from build123d import *

# Parameters (mm, degrees)
BOSS_EXTRUDE1_DEPTH = 10
SKETCH4_W           = 60
SKETCH4_H           = 60
BOSS_EXTRUDE2_DEPTH = 10
SKETCH5_W           = 60
SKETCH5_H           = 147
BOSS_EXTRUDE3_DEPTH = 8
SKETCH6_R           = 12.5
CUT_EXTRUDE1_DEPTH  = 72
SKETCH7_R           = 12.5
BOSS_EXTRUDE4_DEPTH = 50


with BuildPart() as part:
    # Sketch2 → Boss-Extrude1 (new body)
    with BuildSketch(Plane.XY.offset(30)):
        with BuildLine():
            Line((0, -80), (30, -80))
            Line((30, -80), (30, 10))
            Line((30, 10), (15, 77))
            ThreePointArc((15, 77), (-7.5, 92.648353456), (-30, 77))
            Line((-30, 77), (-30, -80))
            Line((-30, -80), (0, -80))
        make_face()
    boss_extrude1 = extrude(amount=BOSS_EXTRUDE1_DEPTH)

    # Sketch4 → Boss-Extrude2 (add)
    with BuildSketch(Plane.XZ.offset(80)):
        Rectangle(SKETCH4_W, SKETCH4_H)
    extrude(amount=-BOSS_EXTRUDE2_DEPTH)

    # Mirror3: Boss-Extrude1 across plane
    add(boss_extrude1.mirror(Plane.XY))

    # Sketch5 → Boss-Extrude3 (add)
    with BuildSketch(Plane.ZY.offset(30)):
        with Locations((0, 3.5)):
            Rectangle(SKETCH5_W, SKETCH5_H)
    extrude(amount=-BOSS_EXTRUDE3_DEPTH)

    # Sketch6 → Cut-Extrude1 (cut, symmetric)
    with BuildSketch(Plane.XY):
        with Locations(Location((0, 0, 0), (0, 0, 180))):
            Circle(SKETCH6_R)
    extrude(amount=CUT_EXTRUDE1_DEPTH, both=True, mode=Mode.SUBTRACT)

    # Sketch7 → Boss-Extrude4 (add)
    with BuildSketch(Plane.XZ.offset(80)):
        with Locations(Location((0, 0, 0), (0, 0, 270))):
            Circle(SKETCH7_R)
    extrude(amount=BOSS_EXTRUDE4_DEPTH)


solid = part.part
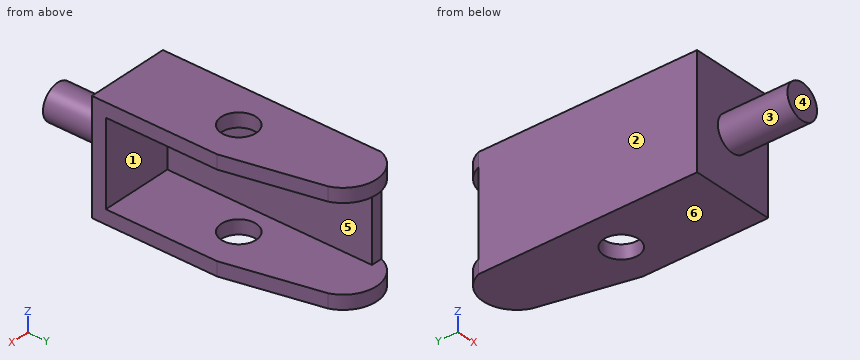
Read the model definition and answer for the solid it produces. Units are mm, in the model's axes. Face numbers are marked on the shaded views. A direction names the side the tool comes from. Coordinates: 2 decimals unless noted, no trailing zeros. Loops run counter-clockwise (first coordinate to the right, second up) from the corner with the lowest first, then second, coordinate; pieces in that order, holes last.
Q1. Each of these flat-tipped pins is pushed along its axis until it touches: pin 1 Ø1 at (x, z) = (-9, 25.5) entering from +Y; pin 2 Ø2 at (y, z) = (-55.5, 16) entering from +X; pin 3 Ø12 at (x, z) = (-6.5, -21) entering from -Y. Where does it stop, or does it pass through?
Q2. Which of the six approach directions +Z, -Z, +X, -X, +Y, -Y give full straight-line access (tool end or side, diameter ignored) to the marked faces 1, 2 and 3?
Q3. The part is cut by section B-B on z = 0. Write down the section's boundary in (x, y), and give its area (3 significant figures).
Q4. The part is cut by section A-A on y = 0. Write down the section's boundary in (x, z).
Q5. The mould has two halves that part along Z. Classify the marked faces 4, 5 and 6: +Z half, -Z half, draft (parallel to the pull), parting line (faces both ways), or undercut.
Q6. The part is cut by section C-C on x = 0. Write down the section's boundary in (y, z), and give its area (3 significant figures).
Q7. Consider probe 1 along Z at (x, y) = (-15.5, 57.5); probe 2 along X at (y, z) = (33.5, 1.5); probe 3 along Y at (x, z) = (25.5, 9). Determine where each line is inside the solid, lowest interval first.
Q8. The part is cut by section D-D on y = -29. Write down the section's boundary in (x, z).
Results below:
1. pin 1: stops at y = -70
1. pin 2: stops at x = -22
1. pin 3: stops at y = -80
2. face 1: +X, +Y
2. face 2: +Z, -Z, -X, +Y, -Y
2. face 3: -Y
3. outline: (-30, -80) - (-12.5, -80) - (-12.5, -130) - (12.5, -130) - (12.5, -80) - (30, -80) - (30, -70) - (-22, -70) - (-22, 77) - (-30, 77) - close
3. area: 3,030 mm2
4. outline: (-30, -40) - (-12.5, -40) - (-12.5, -30) - (-22, -30) - (-22, 30) - (-12.5, 30) - (-12.5, 40) - (-30, 40) - close; (12.5, -40) - (30, -40) - (30, -30) - (12.5, -30) - close; (12.5, 30) - (30, 30) - (30, 40) - (12.5, 40) - close
5. face 4: draft
5. face 5: undercut
5. face 6: -Z half
6. outline: (-130, -12.5) - (-80, -12.5) - (-80, -40) - (-12.5, -40) - (-12.5, -30) - (-70, -30) - (-70, 30) - (-12.5, 30) - (-12.5, 40) - (-80, 40) - (-80, 12.5) - (-130, 12.5) - close; (12.5, -40) - (91.45, -40) - (91.45, -30) - (12.5, -30) - close; (12.5, 30) - (91.45, 30) - (91.45, 40) - (12.5, 40) - close
6. area: 4,780 mm2
7. probe 1: z = -40 to -30, 30 to 40
7. probe 2: x = -30 to -22
7. probe 3: y = -80 to -70
8. outline: (-30, -40) - (30, -40) - (30, -30) - (-22, -30) - (-22, 30) - (30, 30) - (30, 40) - (-30, 40) - close
